```python
from build123d import *

# Parameters (mm, degrees)
SKETCH1_W               = 120
SKETCH1_H               = 100
BOSS_EXTRUDE1_DEPTH     = 100
SKETCH2_W               = 60
SKETCH2_H               = 70
CUT_EXTRUDE2_DEPTH      = 101
CUT_EXTRUDE2_DEPTH_BACK = 1
SKETCH3_R               = 6
CUT_EXTRUDE3_DEPTH      = 51
CUT_EXTRUDE3_DEPTH_BACK = 51
SKETCH5_R               = 4
CUT_EXTRUDE4_DEPTH      = 61
CUT_EXTRUDE4_DEPTH_BACK = 61
SKETCH6_R               = 6
CUT_EXTRUDE5_DEPTH      = 61
CUT_EXTRUDE5_DEPTH_BACK = 61
CUT_EXTRUDE7_START      = -20
SKETCH7_R               = 11
CUT_EXTRUDE7_DEPTH      = 13


with BuildPart() as part:
    # Sketch1 → Boss-Extrude1 (new body)
    with BuildSketch(Plane.XY):
        Rectangle(SKETCH1_W, SKETCH1_H)
    extrude(amount=BOSS_EXTRUDE1_DEPTH)

    # Sketch2 → Cut-Extrude2 (cut, two sides)
    with BuildSketch(Plane.XY) as cut_extrude2_sk:
        Polygon((-60, -20), (-40, -50), (-60, -50), align=None)
        with Locations((0, 15)):
            Rectangle(SKETCH2_W, SKETCH2_H)
        Polygon((60, -50), (40, -50), (60, -20), align=None)
    extrude(amount=CUT_EXTRUDE2_DEPTH, mode=Mode.SUBTRACT)
    extrude(cut_extrude2_sk.sketch, amount=-CUT_EXTRUDE2_DEPTH_BACK, mode=Mode.SUBTRACT)

    # Sketch3 → Cut-Extrude3 (cut, two sides)
    with BuildSketch(Plane(origin=(0, 0, 0), x_dir=(1, 0, 0), z_dir=(0, 1, 0))) as cut_extrude3_sk:
        with Locations((0, -50)):
            Circle(SKETCH3_R)
    extrude(amount=CUT_EXTRUDE3_DEPTH, mode=Mode.SUBTRACT)
    extrude(cut_extrude3_sk.sketch, amount=-CUT_EXTRUDE3_DEPTH_BACK, mode=Mode.SUBTRACT)

    # Sketch5 → Cut-Extrude4 (cut, two sides)
    with BuildSketch(Plane(origin=(0, 0, 0), x_dir=(0, 0, -1), z_dir=(1, 0, 0))) as cut_extrude4_sk:
        with Locations((-91, 15)):
            Circle(SKETCH5_R)
        with Locations((-9, 15)):
            Circle(SKETCH5_R)
    extrude(amount=CUT_EXTRUDE4_DEPTH, mode=Mode.SUBTRACT)
    extrude(cut_extrude4_sk.sketch, amount=-CUT_EXTRUDE4_DEPTH_BACK, mode=Mode.SUBTRACT)

    # Sketch6 → Cut-Extrude5 (cut, two sides)
    with BuildSketch(Plane(origin=(0, 0, 0), x_dir=(0, 0, -1), z_dir=(1, 0, 0))) as cut_extrude5_sk:
        with Locations((-50, 15)):
            Circle(SKETCH6_R)
    extrude(amount=CUT_EXTRUDE5_DEPTH, mode=Mode.SUBTRACT)
    extrude(cut_extrude5_sk.sketch, amount=-CUT_EXTRUDE5_DEPTH_BACK, mode=Mode.SUBTRACT)

    # Sketch7 → Cut-Extrude7 (cut)
    with BuildSketch(Plane(origin=(0, 0, 0), x_dir=(1, 0, 0), z_dir=(0, 1, 0)).offset(CUT_EXTRUDE7_START)):
        with Locations((0, -50)):
            Circle(SKETCH7_R)
    extrude(amount=-CUT_EXTRUDE7_DEPTH, mode=Mode.SUBTRACT)


solid = part.part
```
Model file for the job. Use its own axes, mm. A direction names the side the tool comes from. Round coordinates to 2 decimals unless told otherwise and drop trailing zeros. Order: outer loops, then holes, each group sorted by start corner. A loop starts at its lowest first (then second) coordinate and runs counter-clockwise, first axis right, second up. Notation, with made-up numbers: (28.25, 27) -> (41.25, 27) arc R22 ccw to (41.25, 54) -> close; hole circle Ø3 at (-4, -22). An arc over 180 degrees is marked (long way). Use one line per item in the form item = value.
Item 1: Drill centre lines: line 1 (Z direction, x = 40.5, y = 15); line 2 (X direction, y = 1.5, z = 82.5); line 3 (Z direction, x = 0, y = -24). Where is each one in solid material? Low to high.
Returned:
line_1 = 0 to 5, 13 to 44, 56 to 87, 95 to 100
line_2 = -60 to -30, 30 to 60
line_3 = 0 to 39, 61 to 100
Item 2: Pull direction Y, two halves, no side cores. Call faces 1 (the face through (-44.79, 17.7, 93.95)), 2 (the face through (-45, 50, 49)), 3 (the face through (-60, 7, 49)), 4 (the face through (45, 15, 56)): released by +Y, released by -Y, zero draft, split by the parting line, or undercut.
Returned:
face_1 = undercut
face_2 = released by +Y
face_3 = zero draft
face_4 = undercut
Item 3: Flat gauge pins, fed straight in: pin 1 Ø10 at (y, z) = (-40, 44) entering from +X; pin 2 Ø18 at (x, z) = (0.5, 50) entering from +Y; pin 3 Ø14 at (y, z) = (15, 50) entering from -X; pin 4 Ø10 at (y, z) = (-36, 33.5) entering from -X. Where does each tip first touch, or does it go through?
Returned:
pin_1 = 50
pin_2 = -33
pin_3 = -60
pin_4 = -52.67
Item 4: Cut at C-C, the plane x = 0. Write the cut outline in (y, z).
Returned:
outline = (-50, 0) -> (-20, 0) -> (-20, 39) -> (-33, 39) -> (-33, 44) -> (-50, 44) -> close; (-50, 56) -> (-33, 56) -> (-33, 61) -> (-20, 61) -> (-20, 100) -> (-50, 100) -> close
Item 5: Cut at D-D, the plane y = 15. Give the number of separate pieces and of enclosed holes in the cut face, and give its area (3 significant figures).
Returned:
separate_pieces = 8
enclosed_holes = 0
area = 4,320 mm^2
Item 6: Tool access for faces 5 (the face through (0, -20, 38)), 6 (the face through (60, 7, 49)), 7 (the face through (5, -33, 55)): list every direction of +Z, -Z, +X, -X, +Y, -Y with a clear straight run to the whole face (end or side of a thin tool).
Returned:
face_5 = +Z, -Z, +Y
face_6 = +Z, -Z, +X, +Y, -Y
face_7 = +Y
Item 7: Cut at A-A, the plane y = 25. Write the cut outline in (x, z), and give its area (3 significant figures).
Returned:
outline = (-60, 0) -> (-30, 0) -> (-30, 100) -> (-60, 100) -> close; (30, 0) -> (60, 0) -> (60, 100) -> (30, 100) -> close
area = 6,000 mm^2
Item 8: Cut at B-B, the plane z = 91. Write the cut outline in (x, y).
Returned:
outline = (-60, -20) -> (-40, -50) -> (40, -50) -> (60, -20) -> (60, 11) -> (30, 11) -> (30, -20) -> (-30, -20) -> (-30, 11) -> (-60, 11) -> close; (-60, 19) -> (-30, 19) -> (-30, 50) -> (-60, 50) -> close; (30, 19) -> (60, 19) -> (60, 50) -> (30, 50) -> close
